Geometry: final body of the model. Coordinates: model frame, mm. A direction names the side the tool comes from. Round coordinates to 2 decimals unless told otherwise and drop trailing zeros. Loops run counter-clockwise (first coordinate to the right, second up) from the corner with the lowest first, then second, coordinate; pieces in that order, holes last. Notation, with made-up numbers: (42.5, 56) - (52.5, 56) arc R7 ccw to (52.5, 64) - close; hole circle Ø11 at (-39, -1.75). An arc over 180 degrees is marked (long way). Return JSON: item names as keys, results as strings. Group by question number.
1. Section A-A on z = 17. Return loops of the section in (x, y), and give its area (3 significant figures).
2. Section C-C on y = 77. Return loops of the section in (x, z), and give its area (3 significant figures).
3. First-contact query: pin 1 Ø8 at (x, y) = (24, 24) entering from +Z; pin 2 Ø11.5 at (y, z) = (48.98, 35) entering from -X; pin 3 Ø12 at (x, y) = (24.5, 38.5) entering from +Z; pin 4 Ø3.5 at (y, z) = (48.98, 35) entering from +X. Flat tips, straight axial feed; report the tip coordinate or a pass-through.
4. Draft query along Z for faces 1 (the face through (20, 84, 0)), 2 (the face through (35, 49, 55)), 3 (the face through (34.3, 51, 33)), 4 (the face through (35, 68.981, 22)). Return one class per face: +Z half, -Z half, draft (parallel to the pull), parting line (faces both ways), or undercut.
5. Material intervals for probe 1 along X at (y, z) = (59, 18); probe 2 along Z at (x, y) = (29.5, 19); probe 3 along X at (y, z) = (45, 34), sorted ascending.
6. Set-up query: faces 5 (the face through (30.9, 29.84, 22.32)), 6 (the face through (20, 49, 3)), 7 (the face through (39.145, 68.079, 22.675)), 8 (the face through (39.14, 29.88, 22.32)), 9 (the face through (30, 49, 31)). Return all of +Z, -Z, +X, -X, +Y, -Y with unobstructed straight access to the full face (end or side cutting, diameter ignored); none if empty.
7. Section B-B on x = 18. Return loops of the section in (y, z).
from build123d import *

# Parameters (mm, degrees)
F1_DEPTH     = 10
F3_DEPTH     = 10
F4_R         = 2.25
F5_DEPTH     = 10.001
F6_W         = 40
F6_H         = 3
F7_DEPTH     = 40.001
F8_R         = 4.5
F9_DEPTH     = 5.7
F10_T1_DEPTH = 40
F11_R        = 3


# Not quite as in the source:
# - a fillet or chamfer that OpenCascade refuses, or shapes differently, is made with other operations: its cross-section is extruded or revolved along the edge and cut away or added


with BuildPart() as f1:
    # F0 (on Top) → F1 (new body)
    with BuildSketch(Plane.XY):
        Polygon((0, 100), (0, 0), (40, 0), (40, 96.7579462998), (40, 100), align=None)
    extrude(amount=F1_DEPTH)

    # F2 (on face) → F3 (join)
    with BuildSketch(Plane.YZ.offset(40)):
        with BuildLine():
            Line((28.9808548987, 35), (28.9808548987, 0))
            Line((28.9808548987, 0), (68.9808548987, 0))
            Line((68.9808548987, 0), (68.9808548987, 35))
            ThreePointArc((68.9808548987, 35), (48.9808548987, 55), (28.9808548987, 35))
        make_face()
    extrude(amount=-F3_DEPTH)

    # F4 (on face) → F5 (cut, through all)
    with BuildSketch(Plane(origin=(30, 0, 0), x_dir=(0, -1, 0), z_dir=(-1, 0, 0))):
        with Locations((-48.9808548987, 35)):
            Circle(F4_R)
    extrude(amount=-F5_DEPTH, mode=Mode.SUBTRACT)

    # F6 (on face) → F7 (cut, through all)
    with BuildSketch(Plane.YZ.offset(40)):
        with Locations((48.9808548987, 1.5)):
            Rectangle(F6_W, F6_H)
    extrude(amount=-F7_DEPTH, mode=Mode.SUBTRACT)

    # F8 (on face) → F9 (cut)
    with BuildSketch(Plane.YZ.offset(40)):
        with Locations((48.9808548987, 35)):
            Circle(F8_R)
    extrude(amount=-F9_DEPTH, mode=Mode.SUBTRACT)

    # F10: fillet of radius 8 on 2 edges, made by hand

    # F10_s2 → F10_t1 (join)
    with BuildSketch(Plane.YZ):
        with BuildLine():
            ThreePointArc((68.9808548987, 0), (66.1999585154, 2.2111025509), (62.7358569003, 3))
            Line((62.7358569003, 3), (68.9808548987, 3))
            Line((68.9808548987, 3), (68.9808548987, 0))
        make_face()
        with BuildLine():
            ThreePointArc((35.2258528971, 3), (31.761751282, 2.2111025509), (28.9808548987, 0))
            Line((28.9808548987, 0), (28.9808548987, 3))
            Line((28.9808548987, 3), (35.2258528971, 3))
        make_face()
    extrude(amount=F10_T1_DEPTH)

    # F11
    f11_edges = [f1.edges().sort_by_distance(p)[0] for p in [
        (40, 68.980855, 22.5),
        (30, 68.980855, 22.5),
        (40, 28.980855, 22.5),
        (40, 48.980855, 55),
        (30, 48.980855, 55),
        (30, 28.980855, 22.5),
    ]]
    fillet(f11_edges, radius=F11_R)


solid = f1.part
Taken from the geometry:
{
 "1": {"outline": "(30, 31.98) arc R3 ccw to (33, 28.98) - (37, 28.98) arc R3 ccw to (40, 31.98) - (40, 65.98) arc R3 ccw to (37, 68.98) - (33, 68.98) arc R3 ccw to (30, 65.98) - close", "area": "392 mm2"},
 "2": {"outline": "(0, 0) - (40, 0) - (40, 10) - (0, 10) - close", "area": "400 mm2"},
 "3": {"pin 1": "z = 10", "pin 2": "x = 30", "pin 3": "z = 50.98", "pin 4": "through"},
 "4": {"face 1": "-Z half", "face 2": "+Z half", "face 3": "undercut", "face 4": "draft"},
 "5": {"probe 1": "30 to 40", "probe 2": "0 to 10", "probe 3": "30 to 34.3"},
 "6": {"face 5": "+Z, -X, -Y", "face 6": "-Z, +X, -X", "face 7": "+Z, +X, +Y", "face 8": "+Z, +X, -Y", "face 9": "+Z, -X, +Y, -Y"},
 "7": {"outline": "(0, 0) - (28.98, 0) arc R8 cw to (35.23, 3) - (62.74, 3) arc R8 cw to (68.98, 0) - (100, 0) - (100, 10) - (0, 10) - close"}
}
